from build123d import *

# Parameters (mm, degrees)
F0_R     = 11
F1_DEPTH = 7
F3_R     = 8.5
F4_DEPTH = 4.2


# Not quite as in the source:
# - a feature names something its author has since deleted; it is built from what else it names


with BuildPart() as f1:
    # F0 (on Top) → F1 (new body)
    with BuildSketch(Plane.XY):
        with BuildLine():
            ThreePointArc((9.9944429004, 30.3333333333), (9.9986106286, 30.1666898261), (10, 30))
            ThreePointArc((10, 30), (-0.1666898261, 20.0013893714), (-9.9944429004, 30.3333333333))
            Line((-9.9944429004, 30.3333333333), (-10.7092358725, 8.9014606966))
            ThreePointArc((-10.7092358725, 8.9014606966), (-11.3763303038, 6.5681273633), (-13.0635090303, 4.8237399724))
            Line((-13.0635090303, 4.8237399724), (-31.2666586983, -6.5112252183))
            ThreePointArc((-31.2666586983, -6.5112252183), (-21.1258144232, -6.2576042801), (-15.9807621135, -15))
            ThreePointArc((-15.9807621135, -15), (-17.4050562197, -20.1436629382), (-21.2722157979, -23.8221081151))
            Line((-21.2722157979, -23.8221081151), (-2.3542731578, -13.725200669))
            ThreePointArc((-2.3542731578, -13.725200669), (0, -13.1362547266), (2.3542731578, -13.725200669))
            Line((2.3542731578, -13.725200669), (21.2722157979, -23.8221081151))
            ThreePointArc((21.2722157979, -23.8221081151), (17.3205080757, -10), (31.2666586983, -6.5112252183))
            Line((31.2666586983, -6.5112252183), (13.0635090303, 4.8237399724))
            ThreePointArc((13.0635090303, 4.8237399724), (11.3763303038, 6.5681273633), (10.7092358725, 8.9014606966))
            Line((10.7092358725, 8.9014606966), (9.9944429004, 30.3333333333))
        make_face()
        Circle(F0_R, mode=Mode.SUBTRACT)
        with BuildLine():
            ThreePointArc((-9.9944429004, 30.3333333333), (-0.1666898261, 20.0013893714), (10, 30))
            ThreePointArc((10, 30), (9.9986106286, 30.1666898261), (9.9944429004, 30.3333333333))
            ThreePointArc((9.9944429004, 30.3333333333), (0, 40), (-9.9944429004, 30.3333333333))
        make_face()
        with BuildLine():
            ThreePointArc((-15.9807621135, -15), (-21.1258144232, -6.2576042801), (-31.2666586983, -6.5112252183))
            ThreePointArc((-31.2666586983, -6.5112252183), (-34.6410161514, -20), (-21.2722157979, -23.8221081151))
            ThreePointArc((-21.2722157979, -23.8221081151), (-17.4050562197, -20.1436629382), (-15.9807621135, -15))
        make_face()
        with BuildLine():
            ThreePointArc((35.9807621135, -15), (34.7231578335, -10.1450523096), (31.2666586983, -6.5112252183))
            ThreePointArc((31.2666586983, -6.5112252183), (17.3205080757, -10), (21.2722157979, -23.8221081151))
            ThreePointArc((21.2722157979, -23.8221081151), (31.1244250518, -23.5757058939), (35.9807621135, -15))
        make_face()
    extrude(amount=F1_DEPTH)

    # F3 (on offset) → F4 (cut)
    with BuildSketch(Plane.XY.offset(1.4)):
        with Locations((25.9807621135, -15)):
            Circle(F3_R)
        with Locations((-25.9807621135, -15)):
            Circle(F3_R)
        with Locations((0, 30)):
            Circle(F3_R)
    extrude(amount=F4_DEPTH, mode=Mode.SUBTRACT)


solid = f1.part
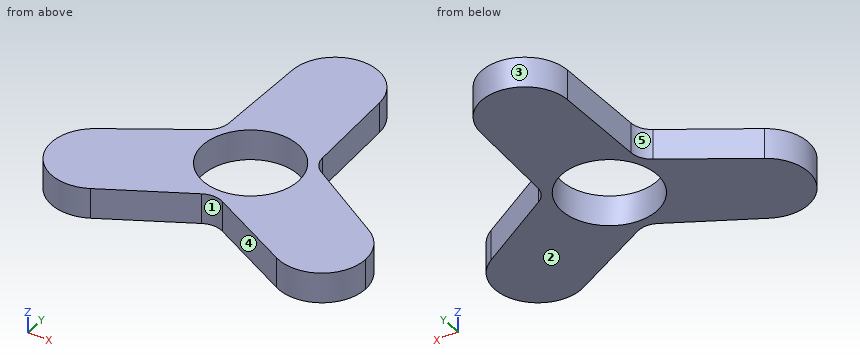
Read the model definition and answer for the solid it produces. Units are mm, in the model's axes. Face numbers are marked on the shaded views. A direction names the side the tool comes from. Give positions to 0.01 mm unless a question says otherwise; leave off trailing zeros. Loops run counter-clockwise (first coordinate to the right, second up) from the corner with the lowest first, then second, coordinate; pieces in that order, holes last. Notation, with made-up numbers: (65.25, -3) -> (91.25, -3) arc R11 cw to (91.25, 10) -> close; hole circle Ø3 at (23, 81.5). An arc over 180 degrees is marked (long way). Answer as CSV lines item,"result".
Item 1: For the marked faces 4 and 5, determine the directions among +Z, -Z, +X, -X, +Y, -Y from which every point of the face is accessible in a straight line to the end or side of a thin tool.
Returned:
face 4,"+Z, -Z, -Y"
face 5,"+Z, -Z, -X, +Y"
Item 2: Each of these flat-tipped pins is pushed along its axis until it touches: pin 1 (2 mm diameter, centred on y = 6.5, z = 2.5, fed in from +X); pin 2 (3 mm diameter, centred on y = 17.5, z = 1, fed in from -X). Where does it stop, or does it pass through?
Returned:
pin 1,"stops at x = 12.2"
pin 2,"stops at x = -10.47"
Item 3: Find section C-C on y = -18.5. Give the vertices of the cut face in (x, z).
Returned:
outline,"(-35.35, 0) -> (-11.3, 0) -> (-11.3, 7) -> (-35.35, 7) -> close; (11.3, 0) -> (35.35, 0) -> (35.35, 7) -> (11.3, 7) -> close; hole (-33.73, 1.4) -> (-18.23, 1.4) -> (-18.23, 5.6) -> (-33.73, 5.6) -> close; hole (18.23, 1.4) -> (33.73, 1.4) -> (33.73, 5.6) -> (18.23, 5.6) -> close"
Item 4: Find section B-B on z = 2.5. Give the vertices of the cut face in (x, y), plus the area to 3 significant figures.
Returned:
outline,"(-31.27, -6.51) arc R10 ccw to (-21.27, -23.82) -> (-2.35, -13.73) arc R5 cw to (2.35, -13.73) -> (21.27, -23.82) arc R10 ccw to (31.27, -6.51) -> (13.06, 4.82) arc R5 cw to (10.71, 8.9) -> (9.99, 30.33) arc R10 ccw to (-9.99, 30.33) -> (-10.71, 8.9) arc R5 cw to (-13.06, 4.82) -> close; hole circle Ø17 at (-25.98, -15); hole circle Ø22 at (0, 0); hole circle Ø17 at (0, 30); hole circle Ø17 at (25.98, -15)"
area,"1,100 mm²"
Item 5: Determine the mould class of the marked faces 1, 2 and 3 for opening direction X: +X half, -X half, draft (parallel to the pull), parting line (faces both ways), or undercut.
Returned:
face 1,"undercut"
face 2,"draft"
face 3,"parting line"
Item 6: Consider line 1 (Y direction, x = 0, z = 4.5); line 2 (Z direction, x = 2, y = 22.5); line 3 (X direction, y = -17.5, z = 4.5). Determine where each line is inside the solid, lowest interval first. Write a range as [from, to].
Returned:
line 1,"y = [-13.14, -11], [11, 21.5], [38.5, 40]"
line 2,"z = [0, 1.4], [5.6, 7]"
line 3,"x = [-35.66, -34.1], [-17.86, -9.43], [9.43, 17.86], [34.1, 35.66]"
Item 7: Find section A-A on x = 0. Give the vertices of the cut face in (y, z).
Returned:
outline,"(-13.14, 0) -> (-11, 0) -> (-11, 7) -> (-13.14, 7) -> close; (11, 0) -> (40, 0) -> (40, 7) -> (11, 7) -> close; hole (21.5, 1.4) -> (38.5, 1.4) -> (38.5, 5.6) -> (21.5, 5.6) -> close"
Item 8: Find section D-D on x = 28. Give the vertices of the cut face in (y, z), plus the area to 3 significant figures.
Returned:
outline,"(-24.79, 0) -> (-4.48, 0) -> (-4.48, 7) -> (-24.79, 7) -> close; hole (-23.26, 1.4) -> (-6.74, 1.4) -> (-6.74, 5.6) -> (-23.26, 5.6) -> close"
area,"72.9 mm²"
